Check sheet for the drawn part. Datum: minimum x, y, z corner. Units: mm. Give positions to 0.01 mm unless a question says otherwise; leave off trailing zeros. Order: outer loops, then holes, each group sorted by start corner. A loop starts at its lowest first (then second) coordinate and runs counter-clockwise, first axis right, second up.
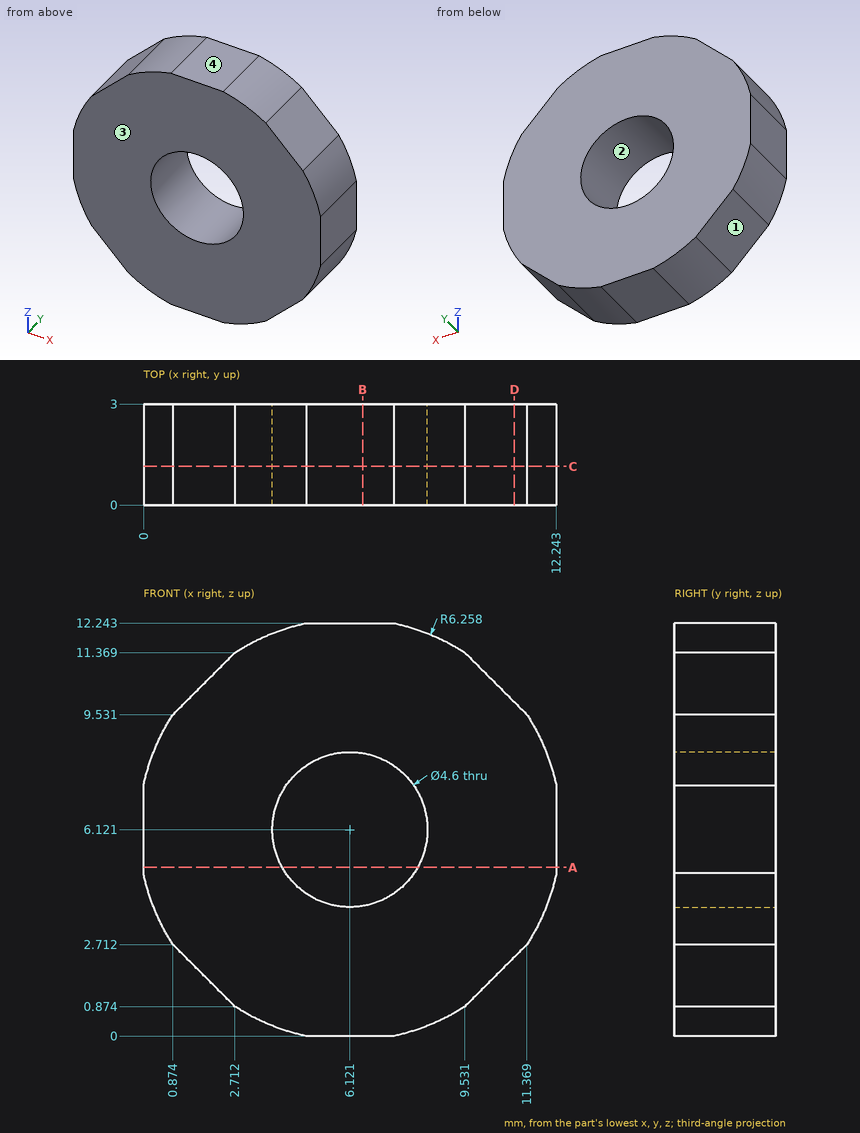
Item 1: Sectioned sample at D-D (x = 11). Enter the section's corners in (y, z).
Reported:
outline: (0, 2.34) - (3, 2.34) - (3, 9.9) - (0, 9.9) - close
Item 2: Sectioned sample at C-C (y = 1.15). Enter the section's corners in (x, z) (1 decimal).
Reported:
outline: (0, 4.8) arc R6.3 ccw to (0.9, 2.7) - (2.7, 0.9) arc R6.3 ccw to (4.8, 0) - (7.4, 0) arc R6.3 ccw to (9.5, 0.9) - (11.4, 2.7) arc R6.3 ccw to (12.2, 4.8) - (12.2, 7.4) arc R6.3 ccw to (11.4, 9.5) - (9.5, 11.4) arc R6.3 ccw to (7.4, 12.2) - (4.8, 12.2) arc R6.3 ccw to (2.7, 11.4) - (0.9, 9.5) arc R6.3 ccw to (0, 7.4) - close; hole circle Ø4.6 at (6.1, 6.1)
Item 3: Sectioned sample at B-B (x = 6.5). Enter the section's corners in (y, z).
Reported:
outline: (0, 0) - (3, 0) - (3, 3.85) - (0, 3.85) - close; (0, 8.39) - (3, 8.39) - (3, 12.24) - (0, 12.24) - close
Item 4: Draft check along Z on the marked faces 1, 2, 3 and 4. Enter one of: released by +Z, released by -Z, zero draft, split by the parting line, or undercut.
Reported:
face 1: released by -Z
face 2: undercut
face 3: zero draft
face 4: released by +Z
Item 5: Sectioned sample at A-A (z = 5). Enter the section's corners in (x, y).
Reported:
outline: (0, 0) - (4.11, 0) - (4.11, 3) - (0, 3) - close; (8.13, 0) - (12.24, 0) - (12.24, 3) - (8.13, 3) - close
Item 6: Scan lines: L1, parallel to Z at x = 6, y = 2.75 (1 decimal); L2, parallel to Z at x = 5.5, y = 1.8 (1 decimal). Record each from-to range of solid material in increasing order.
Reported:
L1: z = 0 to 3.8, 8.4 to 12.2
L2: z = 0 to 3.9, 8.3 to 12.2
Item 7: Gauge pin test, flat ends, axial feed: pin 1 (1.5 mm diameter, centred on y = 1, z = 10, fed in from +X); pin 2 (5 mm diameter, centred on x = 6.5, z = 9.5, fed in from -Y). Record the tip position at first contact, or that the pin passes through.
Reported:
pin 1: stops at x = 11.54
pin 2: stops at y = 0
